Read the model definition and answer for the solid it produces. Units are mm, in the model's axes. Round coordinates to 2 decimals unless told otherwise and drop trailing zeros. Write each loop counter-clockwise with the first axis right and the second up, starting at its lowest first coordinate (ties: lowest second). Pieces come first, ordered by that corner, then holes. Notation, with made-up numbers: (35.5, -32) - (75.5, -32) arc R23 cw to (75.5, -22) - close; hole circle Ø9 at (19.5, -21.75). An arc over 180 degrees is marked (long way). One line per item, written item: value. Start each with the question number.
(1) The mould has two halves that part along Y. Classify faces 1 (the face through (-1, 1, 5)), 2 (the face through (-7.5, -51, 3)), 3 (the face through (72, -34, 3)), 4 (the face through (-64.49, 59.14, 2.46)): +Y half, -Y half, draft (parallel to the pull), parting line (faces both ways), or undercut.
(2) Find the intervals of material crossed by L1, parallel to X at y = 11, z = 4; L2, parallel to X at y = -20.5, z = 0.4; L3, parallel to X at y = 75, z = 1.3, in increasing order.
(3) A cutting plane is placed at C-C, the plane z = 1.4. State how many separate pieces and enclosed holes the cut face has, plus the area to 3 significant figures.
(4) A cutting plane is placed at B-B, the plane x = 31. Determine the outline of the cut face in (y, z).
(5) A cutting plane is placed at A-A, the plane y = 0. Determine the outline of the cut face in (x, z), plus the area to 3 significant figures.
(6) A cutting plane is placed at D-D, the plane x = -77. Determine the outline of the cut face in (y, z).
(7) Flat-ended cylindrical pins translate along their axes: pin 1 Ø1.8 at (x, y) = (25, -75) entering from -Z; pin 2 Ø1.5 at (y, z) = (-51, 2.5) entering from -X; pin 3 Ø1.5 at (y, z) = (57, 1.5) entering from -X; pin 4 Ø2 at (y, z) = (-35.5, 2) entering from +X. Find the tip coordinate at first contact, or state that the pin passes through.
from build123d import *

# Parameters (mm, degrees)
SKETCH_1_R          = 87.5
EXTRUDE_1_DEPTH     = 5
CUT_EXTRUDE_1_DEPTH = 124.844660765
SKETCH_2_R          = 1.5
CUT_EXTRUDE_2_DEPTH = 124.844660765
SKETCH_4_W          = 5
SKETCH_4_H          = 48.25
CUT_EXTRUDE_4_DEPTH = 124.844660765
SKETCH_5_W          = 42
SKETCH_5_H          = 5
SKETCH_5_W_2        = 33.5
CUT_EXTRUDE_7_DEPTH = 124.844660765


with BuildPart() as part:
    # 草圖1 → 填料-伸長1 (new body)
    with BuildSketch(Plane.XY):
        Circle(SKETCH_1_R)
    extrude(amount=EXTRUDE_1_DEPTH)

    # 草圖3 → 除料-伸長1 (cut, through all)
    with BuildSketch(Plane.XY.offset(5)):
        with BuildLine():
            ThreePointArc((-69, -35), (-72.535533906, -33.535533906), (-74, -30))
            Line((-74, -30), (-74, 30))
            ThreePointArc((-74, 30), (-72.535533906, 33.535533906), (-69, 35))
            Line((-69, 35), (-64, 35))
            Line((-64, 35), (-64, -35))
            Line((-64, -35), (-69, -35))
        make_face()
        with BuildLine():
            Line((64, 35), (64, -35))
            Line((64, -35), (69, -35))
            ThreePointArc((69, -35), (72.535533906, -33.535533906), (74, -30))
            Line((74, -30), (74, 30))
            ThreePointArc((74, 30), (72.535533906, 33.535533906), (69, 35))
            Line((69, 35), (64, 35))
        make_face()
    extrude(amount=-CUT_EXTRUDE_1_DEPTH, mode=Mode.SUBTRACT)

    # 草圖2 → 除料-伸長2 (cut, through all)
    with BuildSketch(Plane.XY.offset(5)):
        with Locations((-25, 75)):
            Circle(SKETCH_2_R)
        with Locations(Location((-25, -75, 0), (0, 0, 180))):
            Circle(SKETCH_2_R)
        with Locations(Location((25, 75, 0), (0, 0, 180))):
            Circle(SKETCH_2_R)
        with Locations((25, -75)):
            Circle(SKETCH_2_R)
    extrude(amount=-CUT_EXTRUDE_2_DEPTH, mode=Mode.SUBTRACT)

    # 草圖4 → 除料-伸長4 (cut, through all)
    with BuildSketch(Plane.XY.offset(5)):
        with Locations((43.5, -34.125)):
            Rectangle(SKETCH_4_W, SKETCH_4_H)
        with Locations((43.5, 34.125)):
            Rectangle(SKETCH_4_W, SKETCH_4_H)
        with Locations((-43.5, 34.125)):
            Rectangle(SKETCH_4_W, SKETCH_4_H)
        with Locations((-43.5, -34.125)):
            Rectangle(SKETCH_4_W, SKETCH_4_H)
    extrude(amount=-CUT_EXTRUDE_4_DEPTH, mode=Mode.SUBTRACT)

    # 草圖5 → 除料-伸長7 (cut, through all)
    with BuildSketch(Plane.XY.offset(5)):
        with Locations((-20, 50.75)):
            Rectangle(SKETCH_5_W, SKETCH_5_H)
        with Locations((-24.25, -50.75)):
            Rectangle(SKETCH_5_W_2, SKETCH_5_H)
        with Locations((24.25, -50.75)):
            Rectangle(SKETCH_5_W_2, SKETCH_5_H)
    extrude(amount=-CUT_EXTRUDE_7_DEPTH, mode=Mode.SUBTRACT)


solid = part.part
Here are the results:
1. face 1: draft
1. face 2: undercut
1. face 3: undercut
1. face 4: parting line
2. L1: -86.81 to -74, -64 to -46, -41 to 41, 46 to 64, 74 to 86.81
2. L2: -85.06 to -74, -64 to -46, -41 to 41, 46 to 64, 74 to 85.06
2. L3: -45.07 to -26.5, -23.5 to 23.5, 26.5 to 45.07
3. separate pieces: 1
3. enclosed holes: 10
3. area: 21,100 mm²
4. outline: (-81.82, 0) - (-53.25, 0) - (-53.25, 5) - (-81.82, 5) - close; (-48.25, 0) - (81.82, 0) - (81.82, 5) - (-48.25, 5) - close
5. outline: (-87.5, 0) - (-74, 0) - (-74, 5) - (-87.5, 5) - close; (-64, 0) - (64, 0) - (64, 5) - (-64, 5) - close; (74, 0) - (87.5, 0) - (87.5, 5) - (74, 5) - close
5. area: 775 mm²
6. outline: (-41.56, 0) - (41.56, 0) - (41.56, 5) - (-41.56, 5) - close
7. pin 1: through
7. pin 2: x = -71.63
7. pin 3: x = -67.02
7. pin 4: x = 80.41
